```python
from build123d import *

# Parameters (mm, degrees)
SKETCH1_W                    = 70
SKETCH1_H                    = 200
BASE_FLANGE1_DEPTH           = 8
EDGE_FLANGE1_STRIP_W         = 62
EDGE_FLANGE1_STRIP_H         = 8
EDGE_FLANGE1_STRIP_CUT_DEPTH = 200
EDGE_FLANGE1_DEPTH           = 200
SKETCH9_R                    = 1060
CUT_EXTRUDE1_DEPTH           = 10
SKETCH10_R                   = 9
CUT_EXTRUDE2_DEPTH           = 10


# Sheet-metal steps are written as plain solids
with BuildPart() as part:
    # Sketch1 → Base-Flange1 (new body)
    with BuildSketch(Plane(origin=(0, 0, 0), x_dir=(0, 0, -1), z_dir=(1, 0, 0))):
        Rectangle(SKETCH1_W, SKETCH1_H)
    extrude(amount=-BASE_FLANGE1_DEPTH)

    # Edge-Flange1 strip (across the edge) → Edge-Flange1 strip cut (cut)
    with BuildSketch(Plane(origin=(-8, -100, 35), x_dir=(0, 0, -1), z_dir=(0, 1, 0))):
        with Locations((-8, -4)):
            Rectangle(EDGE_FLANGE1_STRIP_W, EDGE_FLANGE1_STRIP_H)
    extrude(amount=EDGE_FLANGE1_STRIP_CUT_DEPTH, mode=Mode.SUBTRACT)

    # Edge-Flange1 section (across the edge) → Edge-Flange1 (add)
    with BuildSketch(Plane(origin=(-8, -100, 35), x_dir=(0, 0, -1), z_dir=(0, 1, 0))):
        with BuildLine():
            Line((0, 15), (0, 242))
            Line((0, 242), (8, 242))
            Line((8, 242), (8, 15))
            ThreePointArc((8, 15), (12.393398282, 4.393398282), (23, 0))
            Line((23, 0), (23, -8))
            ThreePointArc((23, -8), (6.736544033, -1.263455967), (0, 15))
        make_face()
    extrude(amount=EDGE_FLANGE1_DEPTH)

    # Sketch9 → Cut-Extrude1 (cut)
    with BuildSketch(Plane.XY.offset(35)):
        with Locations((-1150, 332)):
            Circle(SKETCH9_R)
    extrude(amount=-CUT_EXTRUDE1_DEPTH, mode=Mode.SUBTRACT)

    # Sketch10 → Cut-Extrude2 (cut)
    with BuildSketch(Plane(origin=(0, 0, 0), x_dir=(0, 0, -1), z_dir=(1, 0, 0))):
        with Locations((10, -70)):
            Circle(SKETCH10_R)
        with Locations((10, 70)):
            Circle(SKETCH10_R)
    extrude(amount=-CUT_EXTRUDE2_DEPTH, mode=Mode.SUBTRACT)


solid = part.part
```
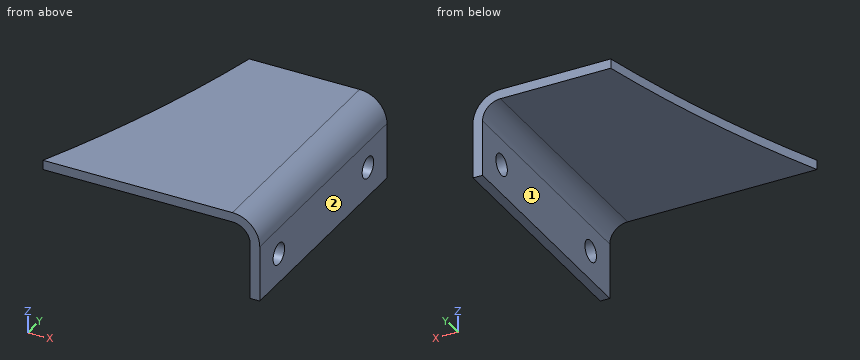
Geometry: final body of the model. Coordinates: model frame, mm. Face numbers are marked on the shaded views. A direction names the side the tool comes from. Round coordinates to 2 decimals unless told otherwise and drop trailing zeros. Write each loop counter-clockwise with the first axis right and the second up, starting at its lowest first coordinate (ties: lowest second). Pieces come first, ordered by that corner, then holes.
Item 1: Set-up query: the marked faces 1 and 2. Return all of +Z, -Z, +X, -X, +Y, -Y with unobstructed straight access to the full face (end or side cutting, diameter ignored); none if empty.
Item 2: Section query B-B (y = 70). Return loops of the section in (x, z).
Item 3: Section query D-D (y = -70). Return loops of the section in (x, z), plus the area to 3 significant figures.
Item 4: Pin query (flat end, axial travel): P1, Ø11, axis at y = 70, z = -10, coming from the +X side; P2, Ø4, axis at x = -118.5, y = 25.5, coming from the -Z side; P3, Ø10, axis at y = 59, z = 24, coming from the +X side; P4, Ø14, axis at y = -9, z = -14.5, coming from the -X side. Return the tip coordinate at first contact, or that it passes through.
Item 5: Material intervals for L1, parallel to Y at x = -4.75, z = -10; L2, parallel to X at y = -34.5, z = -12; L3, parallel to Z at x = -57, y = 84.5, sorted ascending.
Item 6: Section query C-C (x = -72). Return loops of the section in (y, z).
Item 7: Section query A-A (z = -10). Return loops of the section in (x, y).
Completed:
1. face 1: -Z, -X, +Y, -Y
1. face 2: +Z, -Z, +X, +Y, -Y
2. outline: (-122.89, 27) - (-23, 27) arc R15 cw to (-8, 12) - (-8, -1) - (0, -1) - (0, 12) arc R23 ccw to (-23, 35) - (-122.89, 35) - close; (-8, -35) - (0, -35) - (0, -19) - (-8, -19) - close
3. outline: (-169.19, 27) - (-23, 27) arc R15 cw to (-8, 12) - (-8, -1) - (0, -1) - (0, 12) arc R23 ccw to (-23, 35) - (-169.19, 35) - close; (-8, -35) - (0, -35) - (0, -19) - (-8, -19) - close
3. area: 1,640 mm2
4. P1: passes through
4. P2: stops at z = 27
4. P3: stops at x = -1.09
4. P4: stops at x = -8
5. L1: y = -100 to -79, -61 to 61, 79 to 100
5. L2: x = -8 to 0
5. L3: z = 27 to 35
6. outline: (-100, 27) - (100, 27) - (100, 35) - (-100, 35) - close
7. outline: (-8, -100) - (0, -100) - (0, -79) - (-8, -79) - close; (-8, -61) - (0, -61) - (0, 61) - (-8, 61) - close; (-8, 79) - (0, 79) - (0, 100) - (-8, 100) - close
